Geometry: final body of the model. Coordinates: model frame, mm. A direction names the side the tool comes from. Give positions to 0.01 mm unless a question says otherwise; leave off trailing zeros. Write each loop counter-clockwise with the first axis right and the second up, starting at its lowest first coordinate (ties: lowest second). Pieces come first, ordered by that corner, then holes.
from build123d import *


with BuildPart() as part:
    # Sketch1 → Revolve1 (revolve)
    with BuildSketch(Plane.XY):
        with BuildLine():
            Line((-1.5875, 0), (-22.225, 0))
            Line((-22.225, 0), (-22.225, 5.896631452))
            ThreePointArc((-22.225, 5.896631452), (-15.715448212, 21.612079664), (0, 28.121631452))
            Line((0, 28.121631452), (0, 24.946631452))
            Line((0, 24.946631452), (-6.35, 24.946631452))
            Line((-6.35, 24.946631452), (-21.1836, 3.76205518))
            Line((-21.1836, 3.76205518), (-21.1836, 2.1082))
            Line((-21.1836, 2.1082), (-6.35, 2.1082))
            Line((-6.35, 2.1082), (-6.35, 6.35))
            Line((-6.35, 6.35), (-1.5875, 6.35))
            Line((-1.5875, 6.35), (-1.5875, 2.1082))
            Line((-1.5875, 2.1082), (-1.5875, 0))
        make_face()
    revolve(axis=Axis((0, 0, 0), (0, 1, 0)))


solid = part.part
Q1. Pull-direction query (X, two-part tool) for faces 1 (the flat face through (0, 0, -5)), 2 (the cylindrical face through (-21.199, 2.99, 6.676)), 3 (the flat face through (0, 24.947, 0)); classes: released by +X, released by -X, zero draft, split by the parting line, or undercut.
Filled sheet:
face 1: zero draft
face 2: split by the parting line
face 3: undercut
Q2. Ray query, line 1 along X through (y, z) = (3.5, -3); line 2 along Z through (x, y) = (-2.5, 6.25); line 3 along Y through (x, z) = (1.5, 6.5). Return the intervals inside material, ascending.
Filled sheet:
line 1: x = -22.02 to -20.97, -5.6 to 5.6, 20.97 to 22.02
line 2: z = -22.08 to -19.28, -5.84 to 5.84, 19.28 to 22.08
line 3: y = 0 to 2.11, 24.49 to 27.1
Q3. Section D-D on y = 12. Output: boundary loops of the cut face in (x, z).
Filled sheet:
outline: circle Ø42.74 at (0, 0); hole circle Ø30.83 at (0, 0)
Q4. Section C-C on y = 17.5. Output: boundary loops of the cut face in (x, z).
Filled sheet:
outline: circle Ø37.91 at (0, 0); hole circle Ø23.13 at (0, 0)
Q5. Pin query (flat end, axial travel): P1, Ø2, axis at x = -17.5, y = 8.5, coming from the -Z side; P2, Ø1, axis at y = 7.5, z = 17, coming from the +X side; P3, Ø12, axis at x = 13.5, z = -1.5, coming from the +Y side. Return the tip coordinate at first contact, or that it passes through.
Filled sheet:
P1: stops at z = -14.67
P2: stops at x = 14.81
P3: stops at y = 26.79
Q6. Access query for faces 4 (the cylindrical face through (0.34, 3.13, -1.55)), 5 (the cylindrical face through (4.59, 2.92, -20.68)). Directions: +Z, -Z, +X, -X, +Y, -Y. A direction counts if a zero-diameter tool reaches every point of the face in a straight line with its end or side. Return the directions, or none.
Filled sheet:
face 4: -Y
face 5: none
